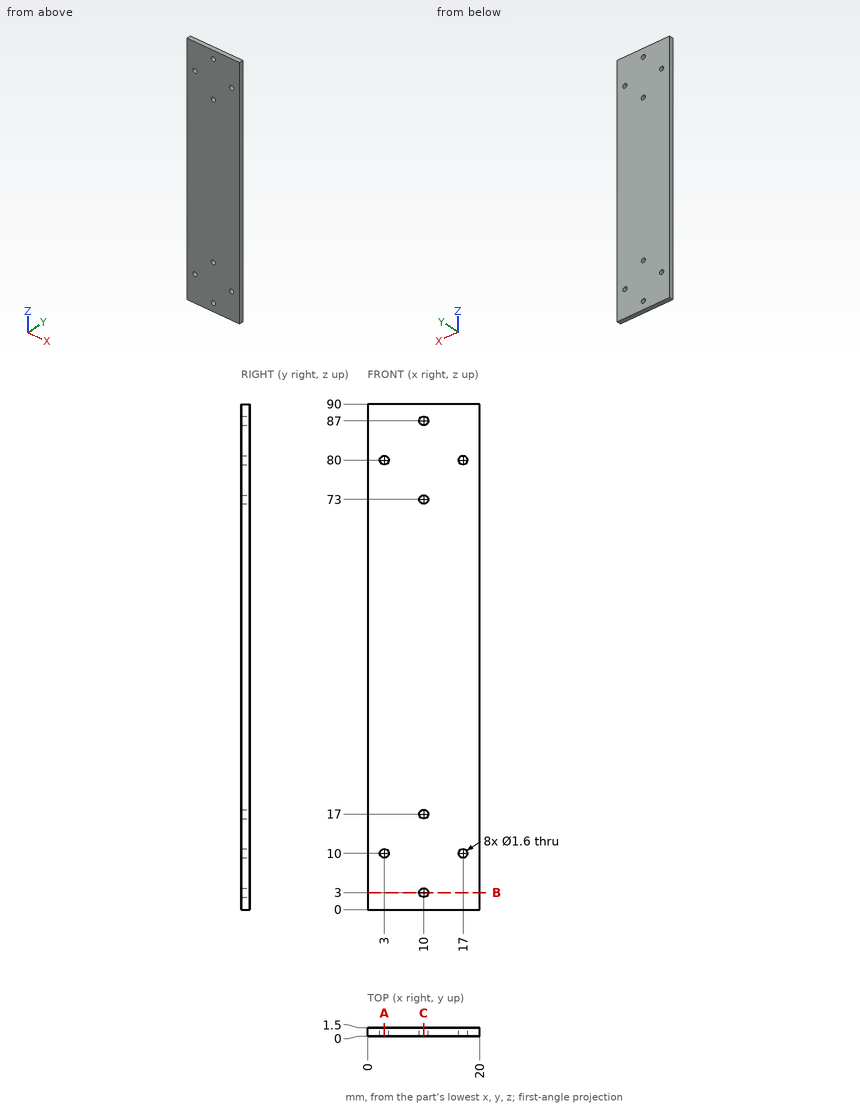
Answer from the drawing. Dimensions are ordinates in mm from the lowest x, y and z of the part. Round coordinates to 2 decimals unless told otherwise and drop trailing zeros. Write each loop counter-clockwise with the first axis right and the second up, starting at its lowest first coordinate (ties: lowest second). Pieces come first, ordered by that corner, then holes.
1. Straight lines are drawn through the part: L1, parallel to Z at x = 17, y = 0.4; L2, parallel to Z at x = 10, y = 1; L3, parallel to X at y = 0.6, z = 10. For each, find the intervals that lie inside material, in ascending order.
2. The part is cut by section A-A, the plane x = 3. Determine the outline of the cut face in (y, z), then the cut area to 3 significant figures.
3. Given pin 1 Ø1 at (x, z) = (3, 10) entering from -Y, flat-ended and moving along its own axis, determine where the tip first touches the part or whether it passes through.
4. The part is cut by section B-B, the plane z = 3. Determine the outline of the cut face in (x, y).
5. The part is cut by section C-C, the plane x = 10. Determine the outline of the cut face in (y, z).
Values:
1. L1: z = 0 to 9.2, 10.8 to 79.2, 80.8 to 90
1. L2: z = 0 to 2.2, 3.8 to 16.2, 17.8 to 72.2, 73.8 to 86.2, 87.8 to 90
1. L3: x = 0 to 2.2, 3.8 to 16.2, 17.8 to 20
2. outline: (0, 0) - (1.5, 0) - (1.5, 9.2) - (0, 9.2) - close; (0, 10.8) - (1.5, 10.8) - (1.5, 79.2) - (0, 79.2) - close; (0, 80.8) - (1.5, 80.8) - (1.5, 90) - (0, 90) - close
2. area: 130 mm2
3. pin 1: passes through
4. outline: (0, 0) - (9.2, 0) - (9.2, 1.5) - (0, 1.5) - close; (10.8, 0) - (20, 0) - (20, 1.5) - (10.8, 1.5) - close
5. outline: (0, 0) - (1.5, 0) - (1.5, 2.2) - (0, 2.2) - close; (0, 3.8) - (1.5, 3.8) - (1.5, 16.2) - (0, 16.2) - close; (0, 17.8) - (1.5, 17.8) - (1.5, 72.2) - (0, 72.2) - close; (0, 73.8) - (1.5, 73.8) - (1.5, 86.2) - (0, 86.2) - close; (0, 87.8) - (1.5, 87.8) - (1.5, 90) - (0, 90) - close
